Here's the drawing with two shaded views (mm, measured from the low corner). I have some questions. A direction names the side the tool comes from. Coordinates: 2 decimals unless noted, no trailing zeros. Loops run counter-clockwise (first coordinate to the right, second up) from the corner with the lowest first, then second, coordinate; pieces in that order, holes last. Notation, with made-up numbers: (51.5, 80) - (69.5, 80) arc R20 cw to (69.5, 102) - close; hole circle Ø5 at (81, 42). An arc over 180 degrees is marked (long way). Use a Markdown table: item, result.
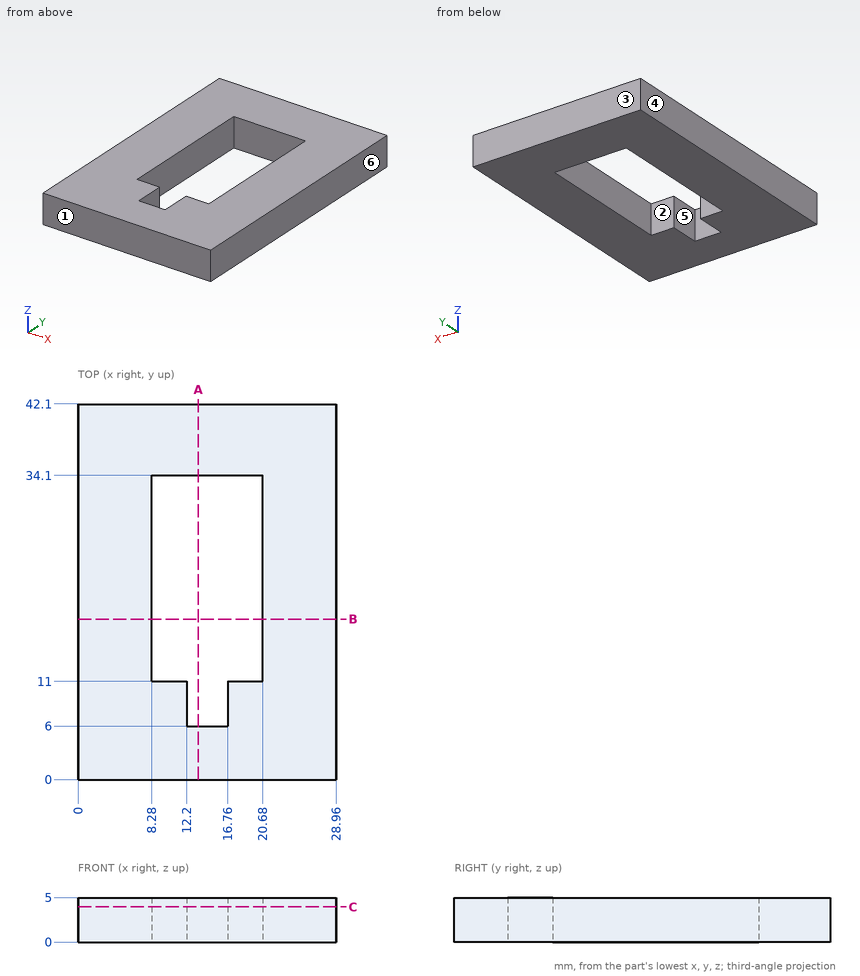
Q1. Which directions (+Z, -Z, +X, -X, +Y, -Y) give clear straight access to the entire face, cutting with the end or side of a thin tool? Please do the marked faces 5 and 6.
Check values:
| item | result |
|---|---|
| face 5 | +Z, -Z |
| face 6 | +Z, -Z, +X, +Y, -Y |
Q2. I want a section at C-C, the plane z = 3.95. Write out the boundary of the cut face in (x, y), then the cut area to 3 significant figures.
Check values:
| item | result |
|---|---|
| outline | (0, 0) - (28.96, 0) - (28.96, 42.1) - (0, 42.1) - close; hole (8.28, 11) - (12.2, 11) - (12.2, 6) - (16.76, 6) - (16.76, 11) - (20.68, 11) - (20.68, 34.1) - (8.28, 34.1) - close |
| area | 910 mm^2 |
Q3. Will this pin go through, and if not, where does the flat tip stop? P1, Ø1, axis at x = 18, y = 33, coming from the -Z side.
Check values:
| item | result |
|---|---|
| P1 | through |
Q4. Please list where these lines run through material, in increasing order: L1, parallel to Y at x = 18.5, z = 0.95; L2, parallel to X at y = 15, z = 1.25; L3, parallel to Y at x = 13.75, z = 2.3. Write a range as from..to.
Check values:
| item | result |
|---|---|
| L1 | 0..11, 34.1..42.1 |
| L2 | 0..8.28, 20.68..28.96 |
| L3 | 0..6, 34.1..42.1 |
Q5. I want a section at A-A, the plane x = 13.5. Write out the boundary of the cut face in (y, z).
Check values:
| item | result |
|---|---|
| outline | (0, 0) - (6, 0) - (6, 5) - (0, 5) - close; (34.1, 0) - (42.1, 0) - (42.1, 5) - (34.1, 5) - close |
Q6. I want a section at B-B, the plane y = 18. Write out the boundary of the cut face in (x, z).
Check values:
| item | result |
|---|---|
| outline | (0, 0) - (8.28, 0) - (8.28, 5) - (0, 5) - close; (20.68, 0) - (28.96, 0) - (28.96, 5) - (20.68, 5) - close |
Q7. If we mould it in two halves opening along Y, with no side actions, what happens to the marked faces 1, 2, 3 and 4? For each: pulls with the +Y half, pulls with the -Y half, needs draft (parallel to the pull), parting line crosses it, or undercut.
Check values:
| item | result |
|---|---|
| face 1 | pulls with the -Y half |
| face 2 | undercut |
| face 3 | pulls with the +Y half |
| face 4 | needs draft |
